Design review of the part built by this model. Coordinates are the model's own, in mm. A direction names the side the tool comes from. Round coordinates to 2 decimals unless told otherwise and drop trailing zeros. Order: outer loops, then holes, each group sorted by start corner. A loop starts at its lowest first (then second) coordinate and runs counter-clockwise, first axis right, second up. Notation, with made-up numbers: (-31.75, -34) - (-18.75, -34) arc R16 cw to (-18.75, -9) - close; hole circle Ø6 at (68, -37). An arc over 180 degrees is marked (long way). Write item = value, one per line.
from build123d import *

# Parameters (mm, degrees)
EXTRUDE_1_DEPTH      = 0.5
EXTRUDE_2_DEPTH      = 4
EXTRUDE_2_DEPTH_BACK = 1
SKETCH_2_R           = 9
SKETCH_3_R           = 7
EXTRUDE_3_DEPTH      = 9
FILLET_1_R           = 0.2
FILLET_2_R           = 0.5
EXTRUDE_4_DEPTH      = 3
EXTRUDE_4_DEPTH_BACK = 3
SKETCH_5_R           = 1
CUT_EXTRUDE_1_DEPTH  = 20
CHAMFER_1_SIZE       = 1.5


with BuildPart() as part:
    # Эскиз1 → Вытянуть1 (new body)
    with BuildSketch(Plane.XY):
        with BuildLine():
            Line((-2.630541488, 14.442307692), (-8.110836255, 4.447115385))
            ThreePointArc((-8.110836255, 4.447115385), (-9.25, 0), (-8.110836255, -4.447115385))
            Line((-8.110836255, -4.447115385), (-2.630541488, -14.442307692))
            ThreePointArc((-2.630541488, -14.442307692), (0, -16), (2.630541488, -14.442307692))
            Line((2.630541488, -14.442307692), (8.110836255, -4.447115385))
            ThreePointArc((8.110836255, -4.447115385), (9.25, 0), (8.110836255, 4.447115385))
            Line((8.110836255, 4.447115385), (2.630541488, 14.442307692))
            ThreePointArc((2.630541488, 14.442307692), (0, 16), (-2.630541488, 14.442307692))
        make_face()
        with BuildLine():
            Line((1.5, 12.5), (1.5, 13.5))
            ThreePointArc((1.5, 13.5), (0, 15), (-1.5, 13.5))
            Line((-1.5, 13.5), (-1.5, 12.5))
            ThreePointArc((-1.5, 12.5), (0, 11), (1.5, 12.5))
        make_face(mode=Mode.SUBTRACT)
        with BuildLine():
            Line((1.5, -12.5), (1.5, -13.5))
            ThreePointArc((1.5, -13.5), (0, -15), (-1.5, -13.5))
            Line((-1.5, -13.5), (-1.5, -12.5))
            ThreePointArc((-1.5, -12.5), (0, -11), (1.5, -12.5))
        make_face(mode=Mode.SUBTRACT)
    extrude(amount=EXTRUDE_1_DEPTH)

    # Эскиз2 → Вытянуть2 (add, two sides: drawn at the far end of the back side and taken through both)
    with BuildSketch(Plane.XY.offset(0.5).offset(-EXTRUDE_2_DEPTH_BACK)):
        Circle(SKETCH_2_R)
    extrude(amount=EXTRUDE_2_DEPTH + EXTRUDE_2_DEPTH_BACK)

    # Эскиз3 → Вытянуть3 (add)
    with BuildSketch(Plane.XY.offset(4.5)):
        Circle(SKETCH_3_R)
    extrude(amount=EXTRUDE_3_DEPTH)

    # Скругление1
    fillet_1_edges = [part.edges().sort_by_distance(p)[0] for p in [
        (-9, 0, 0.5),
        (-9, 0, -0.5),
    ]]
    fillet(fillet_1_edges, radius=FILLET_1_R)

    # Скругление2
    fillet_2_edges = [part.edges().sort_by_distance(p)[0] for p in [
        (-9, 0, 4.5),
        (-7, 0, 4.5),
    ]]
    fillet(fillet_2_edges, radius=FILLET_2_R)

    # Эскиз4 → Вытянуть4 (add, two sides: drawn at the far end of the back side and taken through both)
    with BuildSketch(Plane(origin=(0, 0, 0), x_dir=(0, 0, -1), z_dir=(1, 0, 0)).offset(-EXTRUDE_4_DEPTH_BACK)):
        with BuildLine():
            Line((-22.5, 7.2), (-14.3, 7.2))
            ThreePointArc((-14.3, 7.2), (-13.734314575, 6.965685425), (-13.5, 6.4))
            Line((-13.5, 6.4), (-13.5, 5.184112681))
            Line((-13.5, 5.184112681), (-12.7, 5.184112681))
            Line((-12.7, 5.184112681), (-12.7, 6.4))
            ThreePointArc((-12.7, 6.4), (-13.16862915, 7.53137085), (-14.3, 8))
            Line((-14.3, 8), (-22.5, 8))
            Line((-22.5, 8), (-22.5, 7.2))
        make_face()
        with BuildLine():
            Line((-13.5, -5.184112681), (-13.5, -6.4))
            ThreePointArc((-13.5, -6.4), (-13.734314575, -6.965685425), (-14.3, -7.2))
            Line((-14.3, -7.2), (-22.5, -7.2))
            Line((-22.5, -7.2), (-22.5, -8))
            Line((-22.5, -8), (-14.3, -8))
            ThreePointArc((-14.3, -8), (-13.16862915, -7.53137085), (-12.7, -6.4))
            Line((-12.7, -6.4), (-12.7, -5.184112681))
            Line((-12.7, -5.184112681), (-13.5, -5.184112681))
        make_face()
    extrude(amount=EXTRUDE_4_DEPTH + EXTRUDE_4_DEPTH_BACK)

    # Эскиз5 → Вырез-Вытянуть1 (cut)
    with BuildSketch(Plane.XZ.offset(8)):
        with Locations(Location((0, 19, 0), (0, 0, 270))):
            Circle(SKETCH_5_R)
    extrude(amount=-CUT_EXTRUDE_1_DEPTH, mode=Mode.SUBTRACT)

    # Фаска1
    chamfer_1_edges = [part.edges().sort_by_distance(p)[0] for p in [
        (3, -7.6, 22.5),
        (-3, -7.6, 22.5),
        (3, 7.6, 22.5),
        (-3, 7.6, 22.5),
    ]]
    chamfer(chamfer_1_edges, length=CHAMFER_1_SIZE)


solid = part.part
1) To check wall thickness, follow L1, parallel to X at y = -7.8, z = 19; L2, parallel to Y at x = 1.5, z = 20; L3, parallel to Z at x = -4, y = -9.5. State the ranges of each line that lie inside material, in increasing order. Write a range as from..to.
Findings:
L1 = -3..-1, 1..3
L2 = -8..-7.2, 7.2..8
L3 = 0..0.5
2) We need section D-D on z = 5.5. Write out the cut boundary in (x, y).
Findings:
outline = circle Ø14 at (0, 0)
3) The part is to be moulded in two halves that separate along Z. For faces 1 (the cylindrical face through (-0.04, 7.7, 13.37)), 2 (the flat face through (0, 0, 13.5)), 3 (the flat face through (0, 7.2, 17.5)), say which applies: released by +Z, released by -Z, zero draft, split by the parting line, or undercut.
Findings:
face_1 = undercut
face_2 = released by +Z
face_3 = zero draft
4) For faces 4 (the flat face through (0, -8, 17.5)), 5 (the cylindrical face through (0, 15, 0.2)), 6 (the cylindrical face through (-0.04, -6.96, 13.73)), list the 3-axis set-ups (+Z, -Z, +X, -X, +Y, -Y) from which the entire face can be reached by the end or side of a thin tool; tool diameter is ignored.
Findings:
face_4 = +Z, +X, -X, -Y
face_5 = +Z, -Z
face_6 = +Z, +X, -X
5) Clearance check with flat-ended pins moving along their axes: pin 1 Ø2.5 at (x, z) = (0, 19) entering from +Y; pin 2 Ø0.5 at (y, z) = (7, 18.5) entering from +X; pin 3 Ø12 at (y, z) = (4.5, 7.5) entering from +X. State where each tip first meets the part, or that it passes through.
Findings:
pin_1 = 8
pin_2 = 3
pin_3 = 9
6) We need section B-B on y = 0. Write out the cut boundary in (x, z), and give its area (3 significant figures).
Findings:
outline = (-9.25, 0) - (-9, 0) - (-9, -0.3) arc R0.2 ccw to (-8.8, -0.5) - (8.8, -0.5) arc R0.2 ccw to (9, -0.3) - (9, 0) - (9.25, 0) - (9.25, 0.5) - (9.2, 0.5) arc R0.2 cw to (9, 0.7) - (9, 4) arc R0.5 ccw to (8.5, 4.5) - (7.5, 4.5) arc R0.5 cw to (7, 5) - (7, 13.5) - (-7, 13.5) - (-7, 5) arc R0.5 cw to (-7.5, 4.5) - (-8.5, 4.5) arc R0.5 ccw to (-9, 4) - (-9, 0.7) arc R0.2 cw to (-9.2, 0.5) - (-9.25, 0.5) - close
area = 216 mm^2
7) We need section C-C on y = 12. Write out the cut boundary in (x, z), and give its area (3 significant figures).
Findings:
outline = (-3.97, 0) - (-1.41, 0) - (-1.41, 0.5) - (-3.97, 0.5) - close; (1.41, 0) - (3.97, 0) - (3.97, 0.5) - (1.41, 0.5) - close
area = 2.56 mm^2
8) We need section A-A on z = 19. Write out the cut boundary in (x, y), and give its area (3 significant figures).
Findings:
outline = (-3, -8) - (-1, -8) - (-1, -7.2) - (-3, -7.2) - close; (-3, 7.2) - (-1, 7.2) - (-1, 8) - (-3, 8) - close; (1, -8) - (3, -8) - (3, -7.2) - (1, -7.2) - close; (1, 7.2) - (3, 7.2) - (3, 8) - (1, 8) - close
area = 6.40 mm^2
